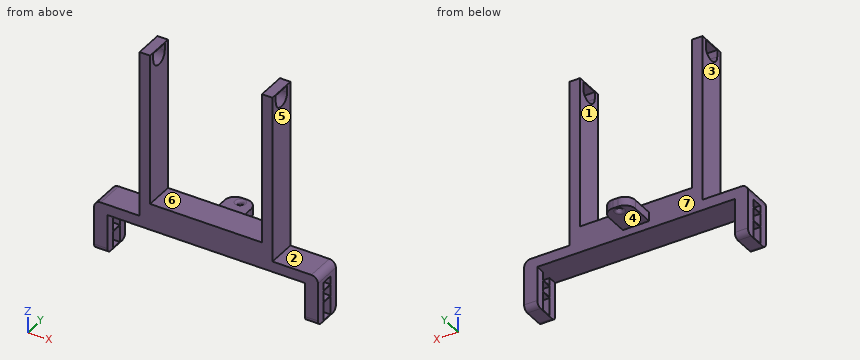
from build123d import *

# Parameters (mm, degrees)
F1_DEPTH  = 22
F2_R      = 5
F4_DEPTH  = 180
F5_W      = 8
F5_H      = 0.5
F6_DEPTH  = 15
F7_W      = 8
F7_H      = 0.5
F8_DEPTH  = 15
F9_R      = 4
F10_W     = 8.5
F10_H     = 30
F11_DEPTH = 195
F12_W     = 20
F12_H     = 6.6774320376
F13_DEPTH = 25
F14_R     = 8
F15_R     = 2
F16_DEPTH = 25
F17_R     = 2
F18_W     = 10
F18_H     = 0.5
F19_DEPTH = 10
F20_W     = 10
F20_H     = 0.5
F21_DEPTH = 9


with BuildPart() as f1:
    # F0 (on Front) → F1 (new body)
    with BuildSketch(Plane.XZ):
        Polygon((-42.5, 0), (-42.5, 115), (-50.5, 115), (-50.5, -12), (0, -12), (50.5, -12), (50.5, 115), (42.5, 115), (42.5, 0), align=None)
        Polygon((0, -12), (-50.5, -12), (-85, -12), (-85, -50), (-75, -50), (-75, -20), (75, -20), (75, -50), (85, -50), (85, -12), (50.5, -12), align=None)
    extrude(amount=F1_DEPTH)

    # F2
    f2_edges = [f1.edges().sort_by_distance(p)[0] for p in [
        (-85, -11, -12),
        (85, -11, -12),
    ]]
    fillet(f2_edges, radius=F2_R)

    # F3 (on face) → F4 (cut)
    with BuildSketch(Plane(origin=(-50.5, 0, 0), x_dir=(0, -1, 0), z_dir=(-1, 0, 0))):
        with BuildLine():
            Line((4.0000428934, 115), (7.2924270352, 115))
            ThreePointArc((7.2924270352, 115), (11, 116.062500298), (14.7075729648, 115))
            Line((14.7075729648, 115), (18.1339288354, 115))
            Line((18.1339288354, 115), (18.1339288354, 118.5624971986))
            Line((18.1339288354, 118.5624971986), (4.0000428934, 118.5624971986))
            Line((4.0000428934, 118.5624971986), (4.0000428934, 115))
        make_face()
        with BuildLine():
            Line((17.9999571066, 109.0870055167), (4.0000428934, 109.0870055167))
            ThreePointArc((4.0000428934, 109.0870055167), (10.9877473719, 102.0625110214), (18, 109.062500298))
            ThreePointArc((18, 109.062500298), (17.9999892766, 109.0747529262), (17.9999571066, 109.0870055167))
        make_face()
        with BuildLine():
            ThreePointArc((7.2924270352, 115), (4.8841455219, 112.4678378735), (4.0000428934, 109.0870055167))
            Line((4.0000428934, 109.0870055167), (17.9999571066, 109.0870055167))
            ThreePointArc((17.9999571066, 109.0870055167), (17.1158544781, 112.4678378735), (14.7075729648, 115))
            Line((14.7075729648, 115), (7.2924270352, 115))
        make_face()
        with BuildLine():
            ThreePointArc((14.7075729648, 115), (17.1158544781, 112.4678378735), (17.9999571066, 109.0870055167))
            Line((17.9999571066, 109.0870055167), (18.1339288354, 109.0870055167))
            Line((18.1339288354, 109.0870055167), (18.1339288354, 115))
            Line((18.1339288354, 115), (14.7075729648, 115))
        make_face()
        with BuildLine():
            Line((4.0000428934, 115), (4.0000428934, 109.0870055167))
            ThreePointArc((4.0000428934, 109.0870055167), (4.8841455219, 112.4678378735), (7.2924270352, 115))
            Line((7.2924270352, 115), (4.0000428934, 115))
        make_face()
    extrude(amount=-F4_DEPTH, mode=Mode.SUBTRACT)

    # F5 (on face) → F6 (join)
    with BuildSketch(Plane.XZ.offset(4.0000428934)):
        with Locations((-46.5, 114.75)):
            Rectangle(F5_W, F5_H)
    extrude(amount=F6_DEPTH)

    # F7 (on face) → F8 (join)
    with BuildSketch(Plane.XZ.offset(4.0000428934)):
        with Locations((46.5, 114.75)):
            Rectangle(F7_W, F7_H)
    extrude(amount=F8_DEPTH)

    # F9
    f9_edges = [f1.edges().sort_by_distance(p)[0] for p in [
        (-80, -22, -50),
        (-80, 0, -50),
        (80, -22, -50),
        (80, 0, -50),
    ]]
    fillet(f9_edges, radius=F9_R)

    # F10 (on face) → F11 (cut)
    with BuildSketch(Plane(origin=(-85, 0, 0), x_dir=(0, -1, 0), z_dir=(-1, 0, 0))):
        with Locations((10.98183, -35)):
            Rectangle(F10_W, F10_H)
    extrude(amount=-F11_DEPTH, mode=Mode.SUBTRACT)

    # F12 (on face) → F13 (join)
    with BuildSketch(Plane(origin=(0, 0, 0), x_dir=(-1, 0, 0), z_dir=(0, 1, 0))):
        with Locations((0, -10.9657765897)):
            Rectangle(F12_W, F12_H)
    extrude(amount=F13_DEPTH)

    # F14
    f14_edges = [f1.edges().sort_by_distance(p)[0] for p in [
        (10, 25, -10.965777),
        (-10, 25, -10.965777),
    ]]
    fillet(f14_edges, radius=F14_R)

    # F15 (on face) → F16 (cut)
    with BuildSketch(Plane.XY.offset(-7.6270605709)):
        with Locations((0, 20)):
            Circle(F15_R)
    extrude(amount=-F16_DEPTH, mode=Mode.SUBTRACT)

    # F17
    f17_edges = [f1.edges().sort_by_distance(p)[0] for p in [
        (-2, 20, -7.627061),
        (-2, 20, -14.304493),
    ]]
    fillet(f17_edges, radius=F17_R)

    # F18 (on face) → F19 (join)
    with BuildSketch(Plane(origin=(0, -15.23183, 0), x_dir=(-1, 0, 0), z_dir=(0, 1, 0))):
        with Locations((-80, -26.3965432942)):
            Rectangle(F18_W, F18_H)
        with Locations((-80, -49.75)):
            Rectangle(F18_W, F18_H)
        with Locations((-80, -35.25)):
            Rectangle(F18_W, F18_H)
    extrude(amount=F19_DEPTH)

    # F20 (on face) → F21 (join)
    with BuildSketch(Plane(origin=(0, -15.23183, 0), x_dir=(-1, 0, 0), z_dir=(0, 1, 0))):
        with Locations((80.0000029802, -26.1500017196)):
            Rectangle(F20_W, F20_H)
        with Locations((80, -49.75)):
            Rectangle(F20_W, F20_H)
        with Locations((80, -36.490347743)):
            Rectangle(F20_W, F20_H)
    extrude(amount=F21_DEPTH)


solid = f1.part
Input: part model. Units: mm. Frame: model coordinates. Face numbers are marked on the shaded views. A direction names the side the tool comes from. Coordinates: 2 decimals unless noted, no trailing zeros. Order: outer loops, then holes, each group sorted by start corner. A loop starts at its lowest first (then second) coordinate and runs counter-clockwise, first axis right, second up. Notation, with made-up numbers: M 32.25,19 L 50.25,19 A18 ccw 50.25,43 Z; hole C 64.5,-21 d4. An arc over 180 degrees is marked long. Answer as CSV lines item,"result".
1. First-contact query: P1, Ø17.5, axis at y = -9, z = 47, coming from the +X side; P2, Ø6.5, axis at y = -15, z = 69, coming from the -X side; P3, Ø1, axis at x = 6, y = 18.5, coming from the +Z side; P4, Ø3, axis at x = -41.5, z = 46, coming from the -Y side. Flat tips, straight axial feed; report the tip coordinate or a pass-through.
Reported:
P1,"x = 50.5"
P2,"x = -50.5"
P3,"z = -7.63"
P4,"y = -22"
2. Section B-B (x = 0). Return the cut outline in (y, z), then the cut area to 3 significant figures.
Reported:
outline,"M -22,-20 L 0,-20 L 0,-14.3 L 16,-14.3 A2 ccw 18,-12.3 L 18,-9.63 A2 ccw 16,-7.63 L 0,-7.63 L 0,0 L -22,0 Z; M 22,-12.3 A2 ccw 24,-14.3 L 25,-14.3 L 25,-7.63 L 24,-7.63 A2 ccw 22,-9.63 Z"
area,"577 mm2"
3. Section D-D (y = -11). State how many separate pieces and enclosed holes the cut face has, then the cut area to 3 significant figures.
Reported:
separate pieces,"9"
enclosed holes,"0"
area,"4,230 mm2"
4. Section A-A (z = 45.5). Return the cut outline in (x, y).
Reported:
outline,"M -50.5,-22 L -42.5,-22 L -42.5,0 L -50.5,0 Z; M 42.5,-22 L 50.5,-22 L 50.5,0 L 42.5,0 Z"
5. Access query for the marked faces 1, 2, 3 and 4. Directions: +Z, -Z, +X, -X, +Y, -Y. A direction counts if a zero-diameter tool reaches every point of the face in a straight line with its end or side. Return the directions, or none.
Reported:
face 1,"+Z, +Y, -Y"
face 2,"+Z, +X, +Y, -Y"
face 3,"+Z, -X, +Y, -Y"
face 4,"-Z, +X, -X, +Y"
6. Pull-direction query (X, two-part tool) for the marked faces 5, 6 and 7; classes: released by +X, released by -X, zero draft, split by the parting line, or undercut.
Reported:
face 5,"released by +X"
face 6,"undercut"
face 7,"zero draft"
7. Material intervals for line 1 (X direction, y = -6.5, z = 51); line 2 (Y direction, x = 0, z = -11.7); line 3 (Z direction, x = 14.5, y = -4), sorted ascending. Write a range as from..to.
Reported:
line 1,"-50.5..-42.5, 42.5..50.5"
line 2,"-22..18, 22..25"
line 3,"-20..0"
8. Section C-C (z = -32). Return the cut outline in (x, y), then the cut area to 3 significant figures.
Reported:
outline,"M -85,-22 L -75,-22 L -75,-15.23 L -85,-15.23 Z; M -85,-6.73 L -75,-6.73 L -75,0 L -85,0 Z; M 75,-22 L 85,-22 L 85,-15.23 L 75,-15.23 Z; M 75,-6.73 L 85,-6.73 L 85,0 L 75,0 Z"
area,"270 mm2"
